Source: three-view drawing plus pictorial views. Frame: mm from the lowest corner of the part. A direction names the side the tool comes from. Give positions to 0.01 mm unless a question says otherwise; leave off trailing zeros. Order: outer loops, then holes, each group sorted by start corner. A loop starts at its lowest first (then second) coordinate and runs counter-clockwise, first axis right, second up.
1) Material intervals for line 1 (Z direction, x = 10, y = 2.1); line 2 (Z direction, x = 11, y = 1.5); line 3 (Y direction, x = 1.5, z = 12.5), sorted ascending.
2) Access query for the marked faces 1 and 2. Directions: +Z, -Z, +X, -X, +Y, -Y. A direction counts if a zero-diameter tool reaches every point of the face in a straight line with its end or side. Return the directions, or none.
3) Section B-B, the plane y = 14.5. Return loops of the section in (x, z), plus the area to 3 significant figures.
4) First-contact query: P1, Ø6, axis at y = 10, z = 25, coming from the +X side; P2, Ø2, axis at y = 14.5, z = 14, coming from the -X side; P3, Ø4, axis at x = 9.5, z = 19, coming from the +Y side. Flat tips, straight axial feed; report the tip coordinate or a pass-through.
5) Section A-A, the plane z = 14. Return loops of the section in (x, y), plus the area to 3 significant figures.
6) Section C-C, the plane z = 7.5. Return loops of the section in (x, y), plus the area to 3 significant figures.
7) Section D-D, the plane y = 2. Return loops of the section in (x, z).
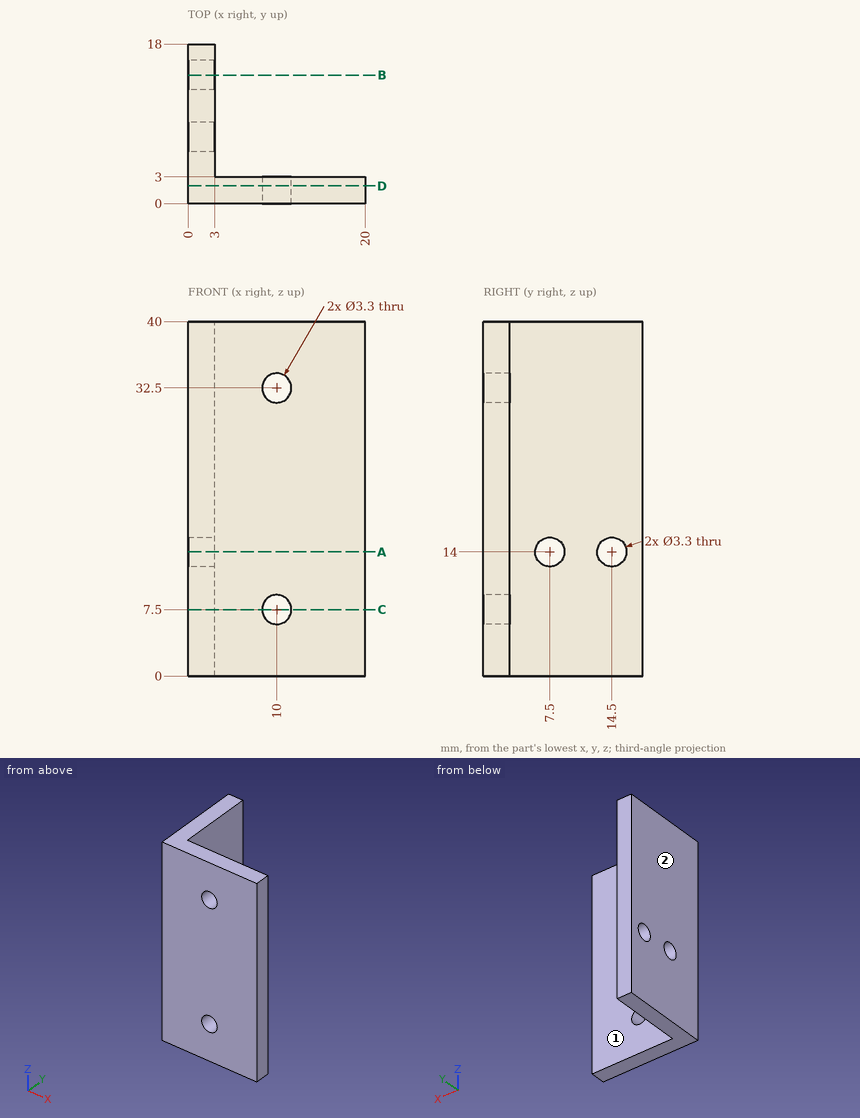
From the geometry:
1. line 1: z = 0 to 5.85, 9.15 to 30.85, 34.15 to 40
1. line 2: z = 0 to 6.19, 8.81 to 31.19, 33.81 to 40
1. line 3: y = 0 to 6.81, 8.19 to 13.81, 15.19 to 18
2. face 1: +Z, -Z, +X, +Y
2. face 2: +Z, -Z, -X, +Y, -Y
3. outline: (0, 0) - (3, 0) - (3, 12.35) - (0, 12.35) - close; (0, 15.65) - (3, 15.65) - (3, 40) - (0, 40) - close
3. area: 110 mm2
4. P1: stops at x = 3
4. P2: passes through
4. P3: stops at y = 3
5. outline: (0, 0) - (20, 0) - (20, 3) - (3, 3) - (3, 5.85) - (0, 5.85) - close; (0, 9.15) - (3, 9.15) - (3, 12.85) - (0, 12.85) - close; (0, 16.15) - (3, 16.15) - (3, 18) - (0, 18) - close
5. area: 85.2 mm2
6. outline: (0, 0) - (8.35, 0) - (8.35, 3) - (3, 3) - (3, 18) - (0, 18) - close; (11.65, 0) - (20, 0) - (20, 3) - (11.65, 3) - close
6. area: 95.1 mm2
7. outline: (0, 0) - (20, 0) - (20, 40) - (0, 40) - close; hole circle Ø3.3 at (10, 7.5); hole circle Ø3.3 at (10, 32.5)
